Source: three-view drawing plus pictorial views. Frame: mm from the lowest corner of the part. Give positions to 0.01 mm unless a question says otherwise; leave off trailing zeros. Loops run counter-clockwise (first coordinate to the right, second up) from the corner with the lowest first, then second, coordinate; pieces in that order, holes last. Notation, with made-up numbers: (-38.5, 2) - (-19.5, 2) arc R20 cw to (-19.5, 24) - close; hole circle Ø10 at (62, 34.5). An arc over 180 degrees is marked (long way). Answer as a JSON object with one key per item and string values. Group by question number.
(1) Material intervals for L1, parallel to X at y = 2.5, z = 1.4; L2, parallel to Z at x = 1.55, y = 11.2; L3, parallel to Y at x = 2.75, z = 2.4, sorted ascending.
(2) Section query B-B (x = 1.55). Return loops of the section in (y, z).
(3) Section query D-D (x = 7.75). Return loops of the section in (y, z), plus the area to 3 significant figures.
(4) Section query A-A (y = 12.25). Return loops of the section in (x, z), plus the area to 3 significant figures.
(5) Section query C-C (z = 0.3). Return loops of the section in (x, y).
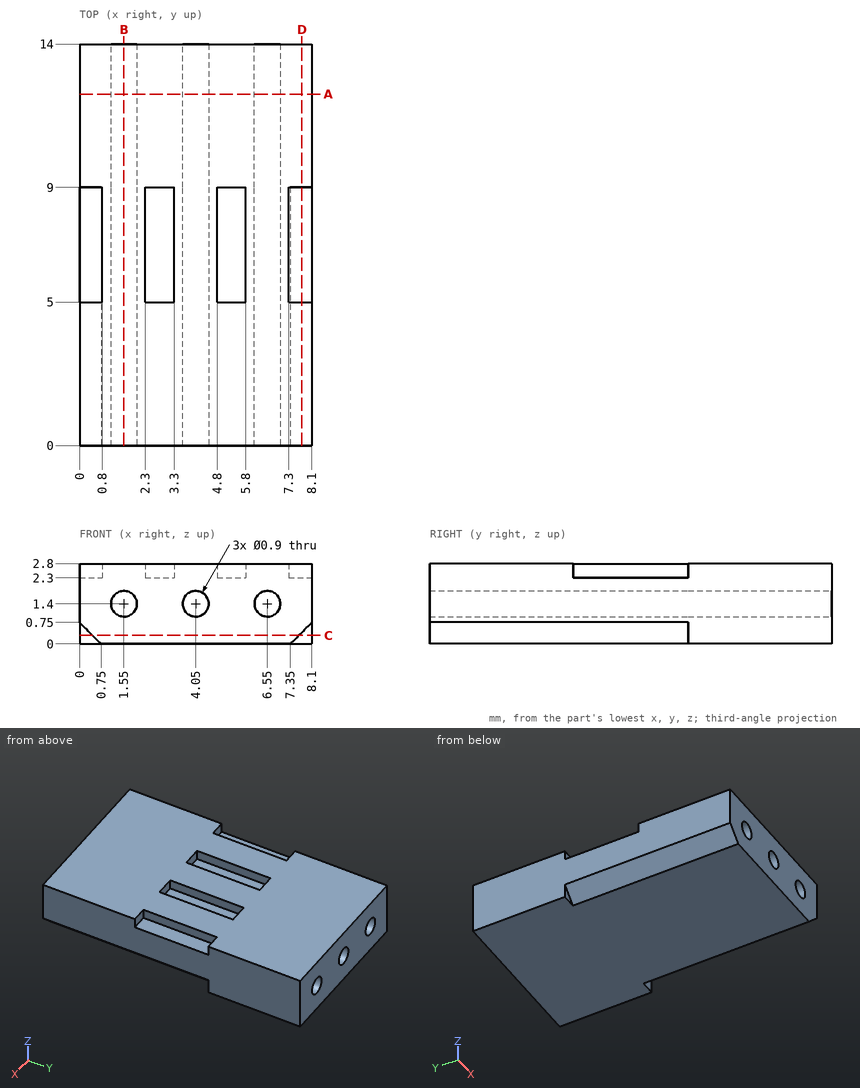
Recorded:
{
 "1": {"L1": "x = 0 to 1.1, 2 to 3.6, 4.5 to 6.1, 7 to 8.1", "L2": "z = 0 to 0.95, 1.85 to 2.8", "L3": "y = 0 to 5, 9 to 14"},
 "2": {"outline": "(0, 0) - (14, 0) - (14, 0.95) - (0, 0.95) - close; (0, 1.85) - (14, 1.85) - (14, 2.8) - (0, 2.8) - close"},
 "3": {"outline": "(0, 0.4) - (9, 0.4) - (9, 0) - (14, 0) - (14, 2.8) - (9, 2.8) - (9, 2.3) - (5, 2.3) - (5, 2.8) - (0, 2.8) - close", "area": "33.6 mm^2"},
 "4": {"outline": "(0, 0) - (8.1, 0) - (8.1, 2.8) - (0, 2.8) - close; hole circle Ø0.9 at (1.55, 1.4); hole circle Ø0.9 at (4.05, 1.4); hole circle Ø0.9 at (6.55, 1.4)", "area": "20.8 mm^2"},
 "5": {"outline": "(0, 9) - (0.45, 9) - (0.45, 0) - (7.65, 0) - (7.65, 9) - (8.1, 9) - (8.1, 14) - (0, 14) - close"}
}
